```python
from build123d import *

# Parameters (mm, degrees)
SKETCH1_W                                      = 75
SKETCH1_H                                      = 95
SKETCH1_R                                      = 1
BOSS_EXTRUDE1_DEPTH                            = 5
CSK_FOR_M5_FLAT_HEAD_MACHINE_SCREW1_AT_2_COUNT = 2
CSK_FOR_M5_FLAT_HEAD_MACHINE_SCREW1_AT_2_PITCH = 28.284271247
CSK_FOR_M5_FLAT_HEAD_MACHINE_SCREW1_AT_3_COUNT = 2
CSK_FOR_M5_FLAT_HEAD_MACHINE_SCREW1_AT_3_PITCH = 40
CSK_FOR_M5_FLAT_HEAD_MACHINE_SCREW1_AT_4_COUNT = 2
CSK_FOR_M5_FLAT_HEAD_MACHINE_SCREW1_AT_4_PITCH = 28.284271247
BOSS_EXTRUDE2_DEPTH                            = 5
CSK_FOR_M5_FLAT_HEAD_MACHINE_SCREW2_AT_2_COUNT = 2
CSK_FOR_M5_FLAT_HEAD_MACHINE_SCREW2_AT_2_PITCH = 105
CSK_FOR_M5_FLAT_HEAD_MACHINE_SCREW2_AT_3_COUNT = 2
CSK_FOR_M5_FLAT_HEAD_MACHINE_SCREW2_AT_3_PITCH = 135.092560861
CSK_FOR_M5_FLAT_HEAD_MACHINE_SCREW2_AT_4_COUNT = 2
CSK_FOR_M5_FLAT_HEAD_MACHINE_SCREW2_AT_4_PITCH = 85


with BuildPart() as part:
    # Sketch1 → Boss-Extrude1 (new body)
    with BuildSketch(Plane(origin=(0, 0, 0), x_dir=(0, 1, 0), z_dir=(0, 0, 1))):
        Rectangle(SKETCH1_W, SKETCH1_H)
        with Locations(Location((0, 20, 0), (0, 0, 270))):
            Circle(SKETCH1_R, mode=Mode.SUBTRACT)
        with Locations(Location((20, 0, 0), (0, 0, 270))):
            Circle(SKETCH1_R, mode=Mode.SUBTRACT)
        with Locations(Location((0, -20, 0), (0, 0, 270))):
            Circle(SKETCH1_R, mode=Mode.SUBTRACT)
        with Locations(Location((-20, 0, 0), (0, 0, 270))):
            Circle(SKETCH1_R, mode=Mode.SUBTRACT)
    extrude(amount=BOSS_EXTRUDE1_DEPTH)

    # Sketch2 → CSK for M5 Flat Head Machine Screw1 (revolve, cut)
    with BuildSketch(Plane(origin=(0, 20, 0), x_dir=(0, 1, 0), z_dir=(1, 0, 0))):
        Polygon((0, 0), (0, 5), (2.75, 5), (2.75, 2.45), (5.2, 0), align=None)
    csk_for_m5_flat_head_machine_screw1 = revolve(axis=Axis((0, 20, -6.35), (0, 0, 1)), mode=Mode.SUBTRACT)

    # CSK for M5 Flat Head Machine Screw1 at 2: CSK for M5 Flat Head Machine Screw1 ×2
    with Locations(*[Vector(-0.7071067811865475, -0.7071067811865477, 0) * (i * CSK_FOR_M5_FLAT_HEAD_MACHINE_SCREW1_AT_2_PITCH) for i in range(1, CSK_FOR_M5_FLAT_HEAD_MACHINE_SCREW1_AT_2_COUNT)]):
        add(csk_for_m5_flat_head_machine_screw1, mode=Mode.SUBTRACT)

    # CSK for M5 Flat Head Machine Screw1 at 3: CSK for M5 Flat Head Machine Screw1 ×2
    with Locations(*[(0, -i * CSK_FOR_M5_FLAT_HEAD_MACHINE_SCREW1_AT_3_PITCH, 0) for i in range(1, CSK_FOR_M5_FLAT_HEAD_MACHINE_SCREW1_AT_3_COUNT)]):
        add(csk_for_m5_flat_head_machine_screw1, mode=Mode.SUBTRACT)

    # CSK for M5 Flat Head Machine Screw1 at 4: CSK for M5 Flat Head Machine Screw1 ×2
    with Locations(*[Vector(0.7071067811865478, -0.7071067811865472, 0) * (i * CSK_FOR_M5_FLAT_HEAD_MACHINE_SCREW1_AT_4_PITCH) for i in range(1, CSK_FOR_M5_FLAT_HEAD_MACHINE_SCREW1_AT_4_COUNT)]):
        add(csk_for_m5_flat_head_machine_screw1, mode=Mode.SUBTRACT)

    # Sketch3 → Boss-Extrude2 (add)
    with BuildSketch(Plane.XY.offset(5)):
        with BuildLine():
            ThreePointArc((-45.428932188, 42.5), (-57.5, 47.5), (-52.5, 35.428932188))
            Line((-52.5, 35.428932188), (-52.5, 42.5))
            Line((-52.5, 42.5), (-45.428932188, 42.5))
        make_face()
        with BuildLine():
            Line((-52.5, 42.5), (-52.5, 35.428932188))
            ThreePointArc((-52.5, 35.428932188), (-49.794019499, 35.967185176), (-47.5, 37.5))
            ThreePointArc((-47.5, 37.5), (-45.967185176, 39.794019499), (-45.428932188, 42.5))
            Line((-45.428932188, 42.5), (-52.5, 42.5))
        make_face()
        with BuildLine():
            ThreePointArc((-45.428932188, 42.5), (-45.967185176, 39.794019499), (-47.5, 37.5))
            Line((-47.5, 37.5), (47.5, 37.5))
            ThreePointArc((47.5, 37.5), (45.967185176, 39.794019499), (45.428932188, 42.5))
            Line((45.428932188, 42.5), (-45.428932188, 42.5))
        make_face()
        with BuildLine():
            ThreePointArc((45.428932188, 42.5), (45.967185176, 39.794019499), (47.5, 37.5))
            ThreePointArc((47.5, 37.5), (49.794019499, 35.967185176), (52.5, 35.428932188))
            Line((52.5, 35.428932188), (52.5, 42.5))
            Line((52.5, 42.5), (45.428932188, 42.5))
        make_face()
        with BuildLine():
            ThreePointArc((59.571067812, 42.5), (52.5, 49.571067812), (45.428932188, 42.5))
            Line((45.428932188, 42.5), (52.5, 42.5))
            Line((52.5, 42.5), (52.5, 35.428932188))
            ThreePointArc((52.5, 35.428932188), (57.5, 37.5), (59.571067812, 42.5))
        make_face()
        with BuildLine():
            Line((47.5, 37.5), (47.5, -37.5))
            ThreePointArc((47.5, -37.5), (49.794019499, -35.967185176), (52.5, -35.428932188))
            Line((52.5, -35.428932188), (52.5, 35.428932188))
            ThreePointArc((52.5, 35.428932188), (49.794019499, 35.967185176), (47.5, 37.5))
        make_face()
        with BuildLine():
            ThreePointArc((47.5, -37.5), (45.967185176, -39.794019499), (45.428932188, -42.5))
            Line((45.428932188, -42.5), (52.5, -42.5))
            Line((52.5, -42.5), (52.5, -35.428932188))
            ThreePointArc((52.5, -35.428932188), (49.794019499, -35.967185176), (47.5, -37.5))
        make_face()
        with BuildLine():
            Line((52.5, -42.5), (45.428932188, -42.5))
            ThreePointArc((45.428932188, -42.5), (52.5, -49.571067812), (59.571067812, -42.5))
            ThreePointArc((59.571067812, -42.5), (57.5, -37.5), (52.5, -35.428932188))
            Line((52.5, -35.428932188), (52.5, -42.5))
        make_face()
        with BuildLine():
            ThreePointArc((-47.5, -37.5), (-45.967185176, -39.794019499), (-45.428932188, -42.5))
            Line((-45.428932188, -42.5), (45.428932188, -42.5))
            ThreePointArc((45.428932188, -42.5), (45.967185176, -39.794019499), (47.5, -37.5))
            Line((47.5, -37.5), (-47.5, -37.5))
        make_face()
        with BuildLine():
            Line((-52.5, -35.428932188), (-52.5, -42.5))
            Line((-52.5, -42.5), (-45.428932188, -42.5))
            ThreePointArc((-45.428932188, -42.5), (-45.967185176, -39.794019499), (-47.5, -37.5))
            ThreePointArc((-47.5, -37.5), (-49.794019499, -35.967185176), (-52.5, -35.428932188))
        make_face()
        with BuildLine():
            Line((-45.428932188, -42.5), (-52.5, -42.5))
            Line((-52.5, -42.5), (-52.5, -35.428932188))
            ThreePointArc((-52.5, -35.428932188), (-57.5, -47.5), (-45.428932188, -42.5))
        make_face()
        with BuildLine():
            Line((-52.5, 35.428932188), (-52.5, -35.428932188))
            ThreePointArc((-52.5, -35.428932188), (-49.794019499, -35.967185176), (-47.5, -37.5))
            Line((-47.5, -37.5), (-47.5, 37.5))
            ThreePointArc((-47.5, 37.5), (-49.794019499, 35.967185176), (-52.5, 35.428932188))
        make_face()
    extrude(amount=-BOSS_EXTRUDE2_DEPTH)

    # Sketch5 → CSK for M5 Flat Head Machine Screw2 (revolve, cut)
    with BuildSketch(Plane(origin=(-52.5, 42.5, 5), x_dir=(0, -1, 0), z_dir=(1, 0, 0))):
        Polygon((0, 0), (0, 5), (2.75, 5), (2.75, 2.45), (5.2, 0), align=None)
    csk_for_m5_flat_head_machine_screw2 = revolve(axis=Axis((-52.5, 42.5, 11.35), (0, 0, -1)), mode=Mode.SUBTRACT)

    # CSK for M5 Flat Head Machine Screw2 at 2: CSK for M5 Flat Head Machine Screw2 ×2
    with Locations(*[(i * CSK_FOR_M5_FLAT_HEAD_MACHINE_SCREW2_AT_2_PITCH, 0, 0) for i in range(1, CSK_FOR_M5_FLAT_HEAD_MACHINE_SCREW2_AT_2_COUNT)]):
        add(csk_for_m5_flat_head_machine_screw2, mode=Mode.SUBTRACT)

    # CSK for M5 Flat Head Machine Screw2 at 3: CSK for M5 Flat Head Machine Screw2 ×2
    with Locations(*[Vector(0.7772448707074855, -0.6291982286679645, 0) * (i * CSK_FOR_M5_FLAT_HEAD_MACHINE_SCREW2_AT_3_PITCH) for i in range(1, CSK_FOR_M5_FLAT_HEAD_MACHINE_SCREW2_AT_3_COUNT)]):
        add(csk_for_m5_flat_head_machine_screw2, mode=Mode.SUBTRACT)

    # CSK for M5 Flat Head Machine Screw2 at 4: CSK for M5 Flat Head Machine Screw2 ×2
    with Locations(*[(0, -i * CSK_FOR_M5_FLAT_HEAD_MACHINE_SCREW2_AT_4_PITCH, 0) for i in range(1, CSK_FOR_M5_FLAT_HEAD_MACHINE_SCREW2_AT_4_COUNT)]):
        add(csk_for_m5_flat_head_machine_screw2, mode=Mode.SUBTRACT)


solid = part.part
```
Here's how the part is built. I have some questions about the finished solid (model axes, mm). A direction names the side the tool comes from. Give positions to 0.01 mm unless a question says otherwise; leave off trailing zeros. Order: outer loops, then holes, each group sorted by start corner. A loop starts at its lowest first (then second) coordinate and runs counter-clockwise, first axis right, second up. Notation, with made-up numbers: (69.25, -31.75) -> (109.25, -31.75) arc R15 cw to (109.25, -15.75) -> close; hole circle Ø7 at (49, -3.5). An arc over 180 degrees is marked (long way). Use CSV: the item, a comma, the result in double quotes. Start each with the question number.
Item 1: On a 3-axis mill with a long thin cutter (end or side, diameter ignored), from which of +Z, -Z, +X, -X, +Y, -Y can I reach the whole of each face in a straight line? I mean faces 1 (the flat face through (52.5, 0, 3)), 2 (the conical face through (-55.379, 42.878, 2.703)). Say none if no direction works.
Item 2: I'm going to push flat-ended pins straight in: P1, Ø2, axis at x = -29.5, z = 3, coming from the -Y side; P2, Ø3.5, axis at x = -20, y = 0, coming from the +Z side (1 decimal); P3, Ø6.5, axis at x = -52.5, y = -42.5, coming from the +Z side. Where does each tip first touch, or does it pass through?
Item 3: Suppose I cut it at B-B (y = 0). List the corners of the cut face in (x, z) for me.
Item 4: Thinking about a two-plate mould opening in Y: for faces 3 (the flat face through (-1, -42.5, 3)), 4 (the flat face through (1, 42.5, 3)), 5 (the cylindrical face through (-54.359, -40.473, 1.293)), 6 (the conical face through (-0.1, -22.9, 2.3)), which applies, pulls with the +Y half, pulls with the -Y half, needs draft (parallel to the pull), parting line crosses it, or undercut?
Item 5: Suppose I cut it at C-C (y = -20). List the corners of the cut face in (x, z) for me.
Item 6: If I drill on probe 1 along Y at (x, z) = (0, 3.4); probe 2 along X at (y, z) = (0, 3.5); probe 3 along X at (y, z) = (43, 0.2), over which ranges is the centre line in solid material (lowest first)? Write a range as [from, to].
Item 7: Suppose I cut it at D-D (z = 1.65). Give the number of separate pieces and of enclosed holes in the cut face, and give its area (3 significant figures).
Item 8: Suppose I cut it at A-A (x = 20). List the corners of the cut face in (y, z) for me.
Answer block:
1,face 1,"+Z, -Z, +X"
1,face 2,"+Z"
2,P1,"stops at y = -42.5"
2,P2,"passes through"
2,P3,"stops at z = 3.05"
3,outline,"(-52.5, 0) -> (-25.2, 0) -> (-22.75, 2.45) -> (-22.75, 5) -> (-52.5, 5) -> close; (-17.25, 2.45) -> (-14.8, 0) -> (14.8, 0) -> (17.25, 2.45) -> (17.25, 5) -> (-17.25, 5) -> close; (22.75, 2.45) -> (25.2, 0) -> (52.5, 0) -> (52.5, 5) -> (22.75, 5) -> close"
4,face 3,"pulls with the -Y half"
4,face 4,"pulls with the +Y half"
4,face 5,"undercut"
4,face 6,"undercut"
5,outline,"(-52.5, 0) -> (-5.2, 0) -> (-2.75, 2.45) -> (-2.75, 5) -> (-52.5, 5) -> close; (2.75, 2.45) -> (5.2, 0) -> (52.5, 0) -> (52.5, 5) -> (2.75, 5) -> close"
6,probe 1,"y = [-42.5, -22.75], [-17.25, 17.25], [22.75, 42.5]"
6,probe 2,"x = [-52.5, -22.75], [-17.25, 17.25], [22.75, 52.5]"
6,probe 3,"x = [-59.55, -55.2], [-49.8, -45.45], [45.45, 49.8], [55.2, 59.55]"
7,separate pieces,"1"
7,enclosed holes,"8"
7,area,"9,140 mm^2"
8,outline,"(-42.5, 0) -> (-5.2, 0) -> (-2.75, 2.45) -> (-2.75, 5) -> (-42.5, 5) -> close; (2.75, 2.45) -> (5.2, 0) -> (42.5, 0) -> (42.5, 5) -> (2.75, 5) -> close"
